Could you check a few things on this drawing? It's one solid part, dimensions in mm from its lowest x, y, z. A direction names the side the tool comes from. Give positions to 0.01 mm unless a question says otherwise; leave off trailing zeros. Write each loop counter-clockwise with the first axis right and the second up, starting at its lowest first coordinate (ties: lowest second). Pieces come first, ordered by that corner, then holes.
1. On a 3-axis mill with a long thin cutter (end or side, diameter ignored), from which of +Z, -Z, +X, -X, +Y, -Y can I reach the whole of each face in a straight line? I mean the marked faces 1, 2 and 3. Say none if no direction works.
2. Thinking about a two-plate mould opening in Z: for the marked faces 4, 5 and 6, which applies, pulls with the +Z half, pulls with the -Z half, needs draft (parallel to the pull), parting line crosses it, or undercut?
3. Suppose I cut it at D-D (z = 20.5). Please give me the cut outline in (x, y).
4. If I drill on probe 1 along Z at (x, y) = (95, 5.25); probe 2 along X at (y, z) = (4.75, 7); probe 3 along X at (y, z) = (8.75, 9) (1 decimal), over which ranges is the centre line in solid material (lowest first)?
5. Suppose I cut it at C-C (x = 5). Please give me the cut outline in (y, z).
6. Suppose I cut it at A-A (x = 41.5). Please give me the cut outline in (y, z).
7. I'm going to push flat-ended pins straight in: pin 1 (2.5 mm diameter, centred on y = 4.5, z = 17, fed in from -X); pin 2 (2.5 mm diameter, centred on x = 5, y = 4, fed in from +Z); pin 3 (4.5 mm diameter, centred on y = 6, z = 63.5, fed in from +X). Where does each tip first touch, or does it pass through?
8. Suppose I cut it at B-B (y = 2). Please give me the cut outline in (x, z), and give its area (3 significant figures).
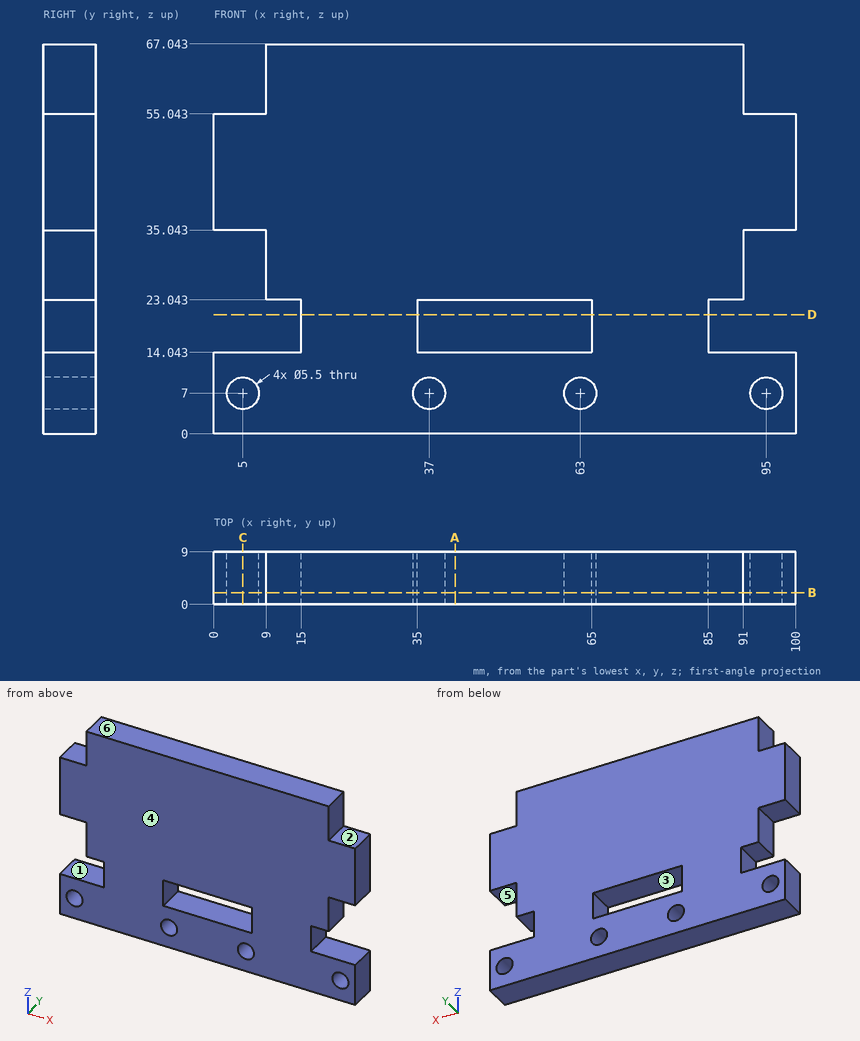
Checks:
1. face 1: -X, +Y, -Y
1. face 2: +Z, +X, +Y, -Y
1. face 3: +Y, -Y
2. face 4: needs draft
2. face 5: undercut
2. face 6: pulls with the +Z half
3. outline: (15, 0) - (35, 0) - (35, 9) - (15, 9) - close; (65, 0) - (85, 0) - (85, 9) - (65, 9) - close
4. probe 1: z = 0 to 4.25, 9.75 to 14.04, 35.04 to 55.04
4. probe 2: x = 0 to 2.25, 7.75 to 34.25, 39.75 to 60.25, 65.75 to 92.25, 97.75 to 100
4. probe 3: x = 0 to 3.1, 6.9 to 35.1, 38.9 to 61.1, 64.9 to 93.1, 96.9 to 100
5. outline: (0, 0) - (9, 0) - (9, 4.25) - (0, 4.25) - close; (0, 9.75) - (9, 9.75) - (9, 14.04) - (0, 14.04) - close; (0, 35.04) - (9, 35.04) - (9, 55.04) - (0, 55.04) - close
6. outline: (0, 0) - (9, 0) - (9, 14.04) - (0, 14.04) - close; (0, 23.04) - (9, 23.04) - (9, 67.04) - (0, 67.04) - close
7. pin 1: stops at x = 15
7. pin 2: stops at z = 55.04
7. pin 3: stops at x = 91
8. outline: (0, 0) - (100, 0) - (100, 14.04) - (85, 14.04) - (85, 23.04) - (91, 23.04) - (91, 35.04) - (100, 35.04) - (100, 55.04) - (91, 55.04) - (91, 67.04) - (9, 67.04) - (9, 55.04) - (0, 55.04) - (0, 35.04) - (9, 35.04) - (9, 23.04) - (15, 23.04) - (15, 14.04) - (0, 14.04) - close; hole circle Ø5.5 at (5, 7); hole circle Ø5.5 at (37, 7); hole (35, 14.04) - (65, 14.04) - (65, 23.04) - (35, 23.04) - close; hole circle Ø5.5 at (63, 7); hole circle Ø5.5 at (95, 7)
8. area: 5,640 mm2
